Part model, mm, in its own coordinate system. Face numbers are marked on the shaded views. A direction names the side the tool comes from. Give positions to 0.01 mm unless a question says otherwise; leave off trailing zeros. Order: outer loops, then holes, each group sorted by start corner. A loop starts at its lowest first (then second) coordinate and runs counter-clockwise, first axis right, second up. Notation, with made-up numbers: (88, 40.5) - (107, 40.5) arc R19 ccw to (107, 48.5) - close; hole circle Ø1 at (-4.5, -11). An arc over 180 degrees is marked (long way). Use a Markdown table: item, result. Add a question column.
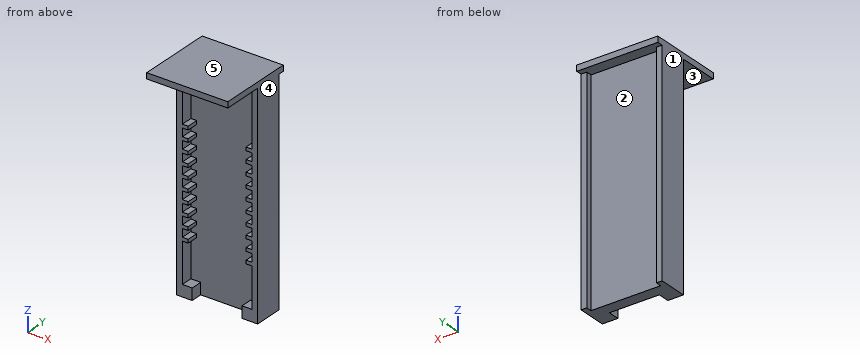
Autodesk Inventor part; units mm, degrees
ref_plane "Work Plane1" through (-10.7426, 6.942, 80.1212) normal (-1, 0, 0) x (0, -1, 0)
ref_plane "YZ Plane" through (0, 0, 0) normal (1, 0, 0) x (0, 1, 0)
ref_plane "XZ Plane" through (0, 0, 0) normal (0, 1, 0) x (-1, 0, 0)
sketch "Sketch1" plane through (0, 0, 0) normal (0, 0, 1) x (1, 0, 0)
  line L0 (-28.5226, 14.562) -> (-28.5226, 1.862)
  line L1 (-28.5226, 1.862) -> (-25.9826, 1.862)
  line L2 (-25.9826, 1.862) -> (-25.9826, 6.942)
  line L3 (-25.9826, 6.942) -> (4.4974, 6.942)
  line L4 (4.4974, 6.942) -> (4.4974, 1.862)
  line L5 (4.4974, 1.862) -> (7.0374, 1.862)
  line L6 (7.0374, 1.862) -> (7.0374, 14.562)
  line L7 (7.0374, 14.562) -> (4.4974, 14.562)
  line L8 (4.4974, 14.562) -> (4.4974, 12.022)
  line L9 (4.4974, 12.022) -> (-25.9826, 12.022)
  line L10 (-25.9826, 12.022) -> (-25.9826, 14.562)
  line L11 (-25.9826, 14.562) -> (-28.5226, 14.562)
  dimension "d0" = 35.56
  dimension "d1" = 2.54
  dimension "d2" = 12.7
  dimension "d3" = 5.08
  dimension "d4" = 2.54
  dimension "d5" = 2.54
extrude "Extrusion1" add sketch "Sketch1" along normal blind 95.25
sketch "Sketch2" plane through (-25.9826, 6.942, 0) normal (0, -1, 0) x (1, 0, 0)
  line L0 (30.48, 95.25) -> (0, 95.25)
  line L1 (0, 69.85) -> (2.54, 69.85)
  line L2 (2.54, 69.85) -> (2.54, 68.326)
  line L3 (2.54, 68.326) -> (0, 68.326)
  line L4 (0, 68.326) -> (0, 69.85)
  line L5 (0, 0) -> (0, 95.25)
  dimension "d8" = 1.524
  dimension "d9" = 2.54
  dimension "d10" = 25.4
extrude "Extrusion2" add sketch "Sketch2" along normal up to surface (5.08 mm away)
pattern_linear "Rectangular Pattern1" count 10 spacing 5.08 along (0, 0, -1) of "Extrusion2"
sketch "Sketch3" plane through (-25.9826, 6.942, 0) normal (0, -1, 0) x (1, 0, 0)
  line L0 (0, 49.53) -> (2.54, 49.53)
  line L1 (2.54, 49.53) -> (2.54, 48.006)
  line L2 (2.54, 48.006) -> (0, 48.006)
  line L3 (0, 44.45) -> (0, 48.006)
  line L4 (0, 44.45) -> (2.54, 44.45)
  line L5 (2.54, 44.45) -> (2.54, 42.926)
  line L6 (2.54, 42.926) -> (0, 42.926)
  line L7 (0, 0) -> (0, 42.926)
  line L8 (0, 0) -> (30.48, 0)
  line L9 (30.48, 0) -> (30.48, 95.25)
  line L10 (30.48, 95.25) -> (0, 95.25)
  line L11 (0, 69.85) -> (0, 95.25)
  line L12 (0, 69.85) -> (2.54, 69.85)
  line L13 (2.54, 69.85) -> (2.54, 68.326)
  line L14 (2.54, 68.326) -> (0, 68.326)
  line L15 (0, 64.77) -> (0, 68.326)
  line L16 (0, 64.77) -> (2.54, 64.77)
  line L17 (2.54, 64.77) -> (2.54, 63.246)
  line L18 (2.54, 63.246) -> (0, 63.246)
  line L19 (0, 59.69) -> (0, 63.246)
  line L20 (0, 59.69) -> (2.54, 59.69)
  line L21 (2.54, 59.69) -> (2.54, 58.166)
  line L22 (2.54, 58.166) -> (0, 58.166)
  line L23 (0, 54.61) -> (0, 58.166)
  line L24 (0, 54.61) -> (2.54, 54.61)
  line L25 (2.54, 54.61) -> (2.54, 53.086)
  line L26 (2.54, 53.086) -> (0, 53.086)
  line L27 (0, 49.53) -> (0, 53.086)
  line L28 (15.24, 80.1212) -> (15.24, 49.6412)
  circle A0 centre (15.24, 64.8812) radius 15.24 construction
  line L29 (30.48, 0) -> (30.48, 95.25)
  line L30 (0, 69.85) -> (0, 95.25)
ref_plane "Work Plane1" through (-10.7426, 6.942, 80.1212) normal (-1, 0, 0) x (0, -1, 0)
sketch "Sketch4" plane through (-25.9826, 6.942, 0) normal (0, -1, 0) x (1, 0, 0)
  line L0 (0, 0) -> (0, 22.606)
  line L1 (0, 0) -> (30.48, 0)
  line L2 (0, 0) -> (5.8186, 0)
  line L3 (0, 5.08) -> (4.318, 5.08)
  line L4 (4.318, 5.08) -> (4.318, 0)
  dimension "d17" = 5.08
  dimension "d18" = 4.318
extrude "Extrusion3" add sketch "Sketch4" along normal up to surface (5.08 mm away)
mirror "Mirror1" about plane through (-10.7426, 6.942, 80.1212) normal (-1, 0, 0) of "Extrusion2", "Rectangular Pattern1"
mirror "Mirror2" about plane through (-10.7426, 6.942, 80.1212) normal (-1, 0, 0) of "Extrusion3"
sketch "Sketch5" plane through (0, 0, 95.25) normal (0, 0, 1) x (1, 0, 0)
  line L0 (-28.5226, 14.562) -> (-25.9826, 14.562)
  line L1 (-28.5226, 1.862) -> (-28.5226, 14.562)
  line L2 (-25.9826, 1.862) -> (-28.5226, 1.862)
  line L3 (-25.9826, 6.942) -> (-25.9826, 1.862)
  line L4 (4.4974, 6.942) -> (-25.9826, 6.942)
  line L5 (4.4974, 1.862) -> (4.4974, 6.942)
  line L6 (7.0374, 1.862) -> (4.4974, 1.862)
  line L7 (7.0374, 14.562) -> (7.0374, 1.862)
  line L8 (4.4974, 14.562) -> (7.0374, 14.562)
  line L9 (4.4974, 12.022) -> (4.4974, 14.562)
  line L10 (-25.9826, 12.022) -> (4.4974, 12.022)
  line L11 (-25.9826, 14.562) -> (-25.9826, 12.022)
  line L12 (-28.5226, 17.102) -> (7.0374, 17.102)
  line L13 (7.0374, 17.102) -> (7.0374, -15.918)
  line L14 (7.0374, -15.918) -> (-28.5226, -15.918)
  line L15 (-28.5226, -15.918) -> (-28.5226, 17.102)
  dimension "d21" = 33.02
  dimension "d22" = 17.78
extrude "Extrusion4" add sketch "Sketch5" along normal blind 2.54
properties part number "slidelat"
1. Drill centre lines: probe 1 along X at (y, z) = (14.5, 14); probe 2 along Y at (x, z) = (-3, 80); probe 3 along Z at (x, y) = (1, 1). Where is each one in solid material? Low to high. Write a range as [from, to].
2. Tool access for the marked faces 1 and 2: list every direction of +Z, -Z, +X, -X, +Y, -Y with a clear straight run to the whole face (end or side of a thin tool).
3. Cut at B-B (x = -20.5). Write the cut outline in (y, z), plus the area to 3 significant figures.
4. Pin check, flat tips, straight feed: P1, Ø1, axis at x = -22.5, z = 43.5, coming from the +Y side; P2, Ø12, axis at x = -6.5, y = 4.5, coming from the -Z side; P3, Ø11.5, axis at x = -18, y = -7.5, coming from the -Z side; P4, Ø6, axis at x = -6.5, z = 41, coming from the -Y side. Stop position of each tip, or through.
5. Cut at A-A (z = 46). Write the cut outline in (x, y), plus the area to 3 significant figures.
6. Cut at C-C (y = -7.5). Write the cut outline in (x, z).
7. Mould opens along X. For the marked faces 3, 4 and 5 say: released by +X, released by -X, zero draft, split by the parting line, or undercut.
Responses:
| question | item | result |
|---|---|---|
| 1 | probe 1 | x = [-28.52, -25.98], [4.5, 7.04] |
| 1 | probe 2 | y = [6.94, 12.02] |
| 1 | probe 3 | z = [95.25, 97.79] |
| 2 | face 1 | +Z, -Z, -X, +Y, -Y |
| 2 | face 2 | -Z, +Y |
| 3 | outline | (-15.92, 95.25) - (6.94, 95.25) - (6.94, 0) - (12.02, 0) - (12.02, 95.25) - (17.1, 95.25) - (17.1, 97.79) - (-15.92, 97.79) - close |
| 3 | area | 568 mm² |
| 4 | P1 | stops at y = 12.02 |
| 4 | P2 | stops at z = 0 |
| 4 | P3 | stops at z = 95.25 |
| 4 | P4 | stops at y = 6.94 |
| 5 | outline | (-28.52, 1.86) - (-25.98, 1.86) - (-25.98, 6.94) - (4.5, 6.94) - (4.5, 1.86) - (7.04, 1.86) - (7.04, 14.56) - (4.5, 14.56) - (4.5, 12.02) - (-25.98, 12.02) - (-25.98, 14.56) - (-28.52, 14.56) - close |
| 5 | area | 219 mm² |
| 6 | outline | (-28.52, 95.25) - (7.04, 95.25) - (7.04, 97.79) - (-28.52, 97.79) - close |
| 7 | face 3 | undercut |
| 7 | face 4 | released by +X |
| 7 | face 5 | zero draft |
